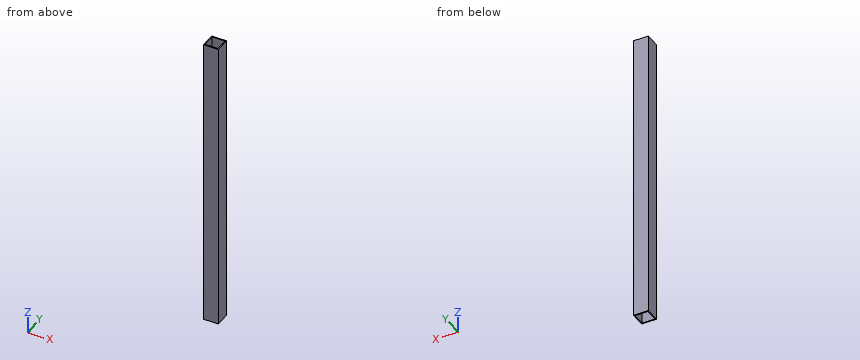
Autodesk Inventor part; units mm, degrees
ref_plane "YZ Plane" through (0, 0, 0) normal (1, 0, 0) x (0, 1, 0)
ref_plane "XZ Plane" through (0, 0, 0) normal (0, 1, 0) x (-1, 0, 0)
ref_plane "XY Plane" through (0, 0, 0) normal (0, 0, 1) x (1, 0, 0)
sketch "スケッチ1" plane through (0, 0, 0) normal (0, 0, 1) x (1, 0, 0)
  line L0 (0, 0) -> (15, 0)
  line L1 (15, 0) -> (15, 15)
  line L2 (15, 15) -> (0, 15)
  line L3 (0, 15) -> (0, 0)
  dimension "d0" = 15
  dimension "d1" = 15
extrude "押し出し1" add sketch "スケッチ1" along normal blind 300
sketch "スケッチ2" plane through (0, 0, 300) normal (0, 0, 1) x (1, 0, 0)
  line L0 (1, 1) -> (14, 1)
  line L1 (14, 1) -> (14, 14)
  line L2 (14, 14) -> (1, 14)
  line L3 (1, 14) -> (1, 1)
  point P0 (0, 0)
  dimension "d4" = 13
  dimension "d5" = 13
extrude "押し出し2" cut sketch "スケッチ2" against normal blind 300
equation "\"BendRadius\" = Thickness"
equation "\"BendReliefWidth\" = Thickness"
equation "\"BendReliefDepth\" = 0.5 * Thickness"
equation "\"CornerReliefSize\" = 4 * Thickness"
equation "\"MinimumRemnant\" = 2 * Thickness"
equation "\"TransitionRadius\" = BendRadius"
equation "\"JacobiRadiusSize\" = BendRadius"
equation "\"GapSize\" = Thickness"
properties part number "0nhk4"
Design review of the part built by this model. Coordinates are the model's own, in mm. Round coordinates to 2 decimals unless told otherwise and drop trailing zeros. Loops run counter-clockwise (first coordinate to the right, second up) from the corner with the lowest first, then second, coordinate; pieces in that order, holes last. Notation, with made-up numbers: (47, 66) - (59, 66) arc R25 ccw to (59, 87) - close; hole circle Ø3 at (-4, 37). An arc over 180 degrees is marked (long way). One line per item, written item: value. Start each with the question number.
1) To check wall thickness, follow L1, parallel to Y at x = 10.5, z = 181. State the ranges of the line that lie inside material, in increasing order. Write a range as from..to.
2) Consider section C-C on z = 248. Give the boundary of the cut face in (x, y).
3) Consider section A-A on x = 5.75. Give the boundary of the cut face in (y, z), then the cut area to 3 significant figures.
Reported:
1. L1: y = 0..1, 14..15
2. outline: (0, 0) - (15, 0) - (15, 15) - (0, 15) - close; hole (1, 1) - (14, 1) - (14, 14) - (1, 14) - close
3. outline: (0, 0) - (1, 0) - (1, 300) - (0, 300) - close; (14, 0) - (15, 0) - (15, 300) - (14, 300) - close
3. area: 600 mm^2
